Could you check a few things on this model? Use its own coordinates, in mm. Give positions to 0.01 mm unless a question says otherwise; leave off trailing zeros. Write each loop counter-clockwise with the first axis right and the second up, starting at its lowest first coordinate (ties: lowest second). Pieces come first, ordered by that corner, then holes. Notation, with made-up numbers: (85, 32) -> (99, 32) arc R13 cw to (99, 37) -> close; hole circle Ø7 at (-19, 19.25). An arc over 180 degrees is marked (long way). One line per question, with ' | ' between items.
from build123d import *

# Parameters (mm, degrees)
CYLINDER1271_R     = 1.5
CYLINDER1271_DEPTH = 100
CYLINDER1270_R     = 1.5
CYLINDER1270_DEPTH = 100
CYLINDER1269_R     = 1.5
CYLINDER1269_DEPTH = 32
CYLINDER1268_R     = 1.5
CYLINDER1268_DEPTH = 32
BOX235_W           = 200
BOX235_H           = 100
BOX235_DEPTH       = 100
BOX233_W           = 200
BOX233_H           = 100
BOX233_DEPTH       = 100
CYLINDER1127_R     = 4
CYLINDER1127_DEPTH = 100
CYLINDER1128_R     = 4
CYLINDER1128_DEPTH = 100
CYLINDER1129_R     = 4
CYLINDER1129_DEPTH = 100
CYLINDER1125_R     = 4
CYLINDER1125_DEPTH = 100
CYLINDER1130_R     = 4
CYLINDER1130_DEPTH = 100
CYLINDER1126_R     = 4
CYLINDER1126_DEPTH = 100
CYLINDER1102_R     = 1.5
CYLINDER1102_DEPTH = 100
CYLINDER1103_R     = 1.5
CYLINDER1103_DEPTH = 100
CYLINDER1104_R     = 1.5
CYLINDER1104_DEPTH = 100
CYLINDER1105_R     = 1.5
CYLINDER1105_DEPTH = 100
CYLINDER1106_R     = 1.5
CYLINDER1106_DEPTH = 100
CYLINDER1107_R     = 1.5
CYLINDER1107_DEPTH = 100
CYLINDER1108_R     = 1.5
CYLINDER1108_DEPTH = 100
CYLINDER1101_R     = 1.5
CYLINDER1101_DEPTH = 100
CYLINDER1092_R     = 59
CYLINDER1092_DEPTH = 4


with BuildPart() as obj1:
    # Cylinder1271 → Cylinder1271 (new body)
    with BuildSketch(Plane(origin=(14, 0, -60), x_dir=(1, 0, 0), z_dir=(0, 0, 1))):
        Circle(CYLINDER1271_R)
    extrude(amount=CYLINDER1271_DEPTH)


with BuildPart() as obj2:
    # Cylinder1270 → Cylinder1270 (new body)
    with BuildSketch(Plane(origin=(90, 0, -60), x_dir=(1, 0, 0), z_dir=(0, 0, 1))):
        Circle(CYLINDER1270_R)
    extrude(amount=CYLINDER1270_DEPTH)

    # Compound834: union obj1
    add(obj1.part)


with BuildPart() as obj3:
    # Cylinder1269 → Cylinder1269 (new body)
    with BuildSketch(Plane(origin=(78, 41, -42), x_dir=(1, 0, 0), z_dir=(0, 0, 1))):
        Circle(CYLINDER1269_R)
    extrude(amount=CYLINDER1269_DEPTH)


with BuildPart() as compound833:
    # Cylinder1268 → Cylinder1268 (new body)
    with BuildSketch(Plane(origin=(26, 41, -42), x_dir=(1, 0, 0), z_dir=(0, 0, 1))):
        Circle(CYLINDER1268_R)
    extrude(amount=CYLINDER1268_DEPTH)

    # Compound833: union obj3
    add(obj3.part)


with BuildPart() as krychle235:
    # Box235 → Box235 (new body)
    with BuildSketch(Plane(origin=(-60, 44, -90), x_dir=(1, 0, 0), z_dir=(0, 0, 1))):
        with Locations((100, 50)):
            Rectangle(BOX235_W, BOX235_H)
    extrude(amount=BOX235_DEPTH)


with BuildPart() as krychle233:
    # Box233 → Box233 (new body)
    with BuildSketch(Plane(origin=(-60, -144, -90), x_dir=(1, 0, 0), z_dir=(0, 0, 1))):
        with Locations((100, 50)):
            Rectangle(BOX233_W, BOX233_H)
    extrude(amount=BOX233_DEPTH)


with BuildPart() as obj4:
    # Cylinder1127 → Cylinder1127 (new body)
    with BuildSketch(Plane(origin=(-36, 34, -90), x_dir=(1, 0, 0), z_dir=(0, 0, 1))):
        Circle(CYLINDER1127_R)
    extrude(amount=CYLINDER1127_DEPTH)


with BuildPart() as obj5:
    # Cylinder1128 → Cylinder1128 (new body)
    with BuildSketch(Plane(origin=(-36, -34, -90), x_dir=(1, 0, 0), z_dir=(0, 0, 1))):
        Circle(CYLINDER1128_R)
    extrude(amount=CYLINDER1128_DEPTH)


with BuildPart() as obj6:
    # Cylinder1129 → Cylinder1129 (new body)
    with BuildSketch(Plane(origin=(50, 0, -90), x_dir=(1, 0, 0), z_dir=(0, 0, 1))):
        Circle(CYLINDER1129_R)
    extrude(amount=CYLINDER1129_DEPTH)


with BuildPart() as obj7:
    # Cylinder1125 → Cylinder1125 (new body)
    with BuildSketch(Plane(origin=(36, 34, -90), x_dir=(1, 0, 0), z_dir=(0, 0, 1))):
        Circle(CYLINDER1125_R)
    extrude(amount=CYLINDER1125_DEPTH)


with BuildPart() as obj8:
    # Cylinder1130 → Cylinder1130 (new body)
    with BuildSketch(Plane(origin=(36, -34, -90), x_dir=(1, 0, 0), z_dir=(0, 0, 1))):
        Circle(CYLINDER1130_R)
    extrude(amount=CYLINDER1130_DEPTH)


with BuildPart() as obj9:
    # Cylinder1126 → Cylinder1126 (new body)
    with BuildSketch(Plane(origin=(-50, 0, -90), x_dir=(1, 0, 0), z_dir=(0, 0, 1))):
        Circle(CYLINDER1126_R)
    extrude(amount=CYLINDER1126_DEPTH)

    # Compound565: union obj4, obj5, obj6, obj7, obj8
    add(obj4.part)
    add(obj5.part)
    add(obj6.part)
    add(obj7.part)
    add(obj8.part)


with BuildPart() as obj10:
    # Cylinder1102 → Cylinder1102 (new body)
    with BuildSketch(Plane(origin=(103, 6, -60), x_dir=(1, 0, 0), z_dir=(0, 0, 1))):
        Circle(CYLINDER1102_R)
    extrude(amount=CYLINDER1102_DEPTH)


with BuildPart() as obj11:
    # Cylinder1103 → Cylinder1103 (new body)
    with BuildSketch(Plane(origin=(76, 18, -60), x_dir=(1, 0, 0), z_dir=(0, 0, 1))):
        Circle(CYLINDER1103_R)
    extrude(amount=CYLINDER1103_DEPTH)


with BuildPart() as obj12:
    # Cylinder1104 → Cylinder1104 (new body)
    with BuildSketch(Plane(origin=(91, -21, -60), x_dir=(1, 0, 0), z_dir=(0, 0, 1))):
        Circle(CYLINDER1104_R)
    extrude(amount=CYLINDER1104_DEPTH)


with BuildPart() as obj13:
    # Cylinder1105 → Cylinder1105 (new body)
    with BuildSketch(Plane(origin=(13, -21, -60), x_dir=(1, 0, 0), z_dir=(0, 0, 1))):
        Circle(CYLINDER1105_R)
    extrude(amount=CYLINDER1105_DEPTH)


with BuildPart() as obj14:
    # Cylinder1106 → Cylinder1106 (new body)
    with BuildSketch(Plane(origin=(28, 18, -60), x_dir=(1, 0, 0), z_dir=(0, 0, 1))):
        Circle(CYLINDER1106_R)
    extrude(amount=CYLINDER1106_DEPTH)


with BuildPart() as obj15:
    # Cylinder1107 → Cylinder1107 (new body)
    with BuildSketch(Plane(origin=(1, -12, -60), x_dir=(1, 0, 0), z_dir=(0, 0, 1))):
        Circle(CYLINDER1107_R)
    extrude(amount=CYLINDER1107_DEPTH)


with BuildPart() as obj16:
    # Cylinder1108 → Cylinder1108 (new body)
    with BuildSketch(Plane(origin=(1, 6, -60), x_dir=(1, 0, 0), z_dir=(0, 0, 1))):
        Circle(CYLINDER1108_R)
    extrude(amount=CYLINDER1108_DEPTH)


with BuildPart() as obj17:
    # Cylinder1101 → Cylinder1101 (new body)
    with BuildSketch(Plane(origin=(103, -12, -60), x_dir=(1, 0, 0), z_dir=(0, 0, 1))):
        Circle(CYLINDER1101_R)
    extrude(amount=CYLINDER1101_DEPTH)

    # Compound562: union obj10, obj11, obj12, obj13, obj14, obj15, obj16
    add(obj10.part)
    add(obj11.part)
    add(obj12.part)
    add(obj13.part)
    add(obj14.part)
    add(obj15.part)
    add(obj16.part)


with BuildPart() as cut291:
    # Cylinder1092 → Cylinder1092 (new body)
    with BuildSketch(Plane(origin=(52, 0, -26), x_dir=(1, 0, 0), z_dir=(0, 0, 1))):
        Circle(CYLINDER1092_R)
    extrude(amount=CYLINDER1092_DEPTH)

    # Cut250: cut obj17
    add(obj17.part, mode=Mode.SUBTRACT)

    # Cut251: cut obj9
    add(obj9.part, mode=Mode.SUBTRACT)

    # Cut285: cut Krychle233
    add(krychle233.part, mode=Mode.SUBTRACT)

    # Cut287: cut Krychle235
    add(krychle235.part, mode=Mode.SUBTRACT)

    # Cut288: cut Compound833
    add(compound833.part, mode=Mode.SUBTRACT)

    # Cut291: cut obj2
    add(obj2.part, mode=Mode.SUBTRACT)


solid = cut291.part
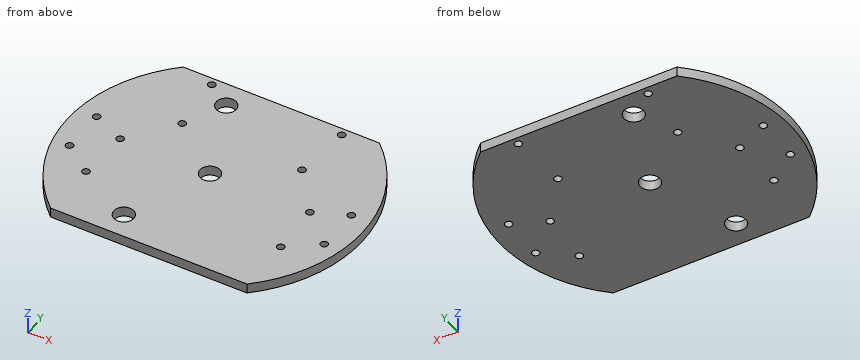
Q1. Imagine slicing it at A-A on y = 0. Please give me the cut outline in (x, z), and give its area (3 significant figures).
Answer below:
outline: (-7, -26) -> (12.5, -26) -> (12.5, -22) -> (-7, -22) -> close; (15.5, -26) -> (46, -26) -> (46, -22) -> (15.5, -22) -> close; (54, -26) -> (88.5, -26) -> (88.5, -22) -> (54, -22) -> close; (91.5, -26) -> (111, -26) -> (111, -22) -> (91.5, -22) -> close | area: 416 mm^2
Q2. If I drill on line 1 along Y through (x, z) = (36, -24.1); line 2 along X through (y, z) = (-21, -24); line 3 along X through (y, z) = (6, -25.2), over which ranges is the centre line in solid material (lowest first)?
Answer below:
line 1: y = -44 to -38, -30 to 30, 38 to 44 | line 2: x = -3.14 to 11.5, 14.5 to 89.5, 92.5 to 107.14 | line 3: x = -6.69 to -0.5, 2.5 to 101.5, 104.5 to 110.69
Q3. Will this pin go through, and if not, where does the flat tip stop? pin 1 (3.5 mm diameter, centred on x = 1, y = -12, fed in from +Z).
Answer below:
pin 1: stops at z = -22
Q4. Imagine slicing it at D-D on y = -21. Please give me the cut outline in (x, z).
Answer below:
outline: (-3.14, -26) -> (11.5, -26) -> (11.5, -22) -> (-3.14, -22) -> close; (14.5, -26) -> (89.5, -26) -> (89.5, -22) -> (14.5, -22) -> close; (92.5, -26) -> (107.14, -26) -> (107.14, -22) -> (92.5, -22) -> close
Q5. Imagine slicing it at C-C on z = -23.15. Count the separate pieces of the cut face and the enclosed holes in it, and give its area (3 significant figures).
Answer below:
separate pieces: 1 | enclosed holes: 15 | area: 9,080 mm^2
Q6. Imagine slicing it at B-B on x = 1. Please give me the cut outline in (y, z), and give its area (3 significant figures).
Answer below:
outline: (-29.66, -26) -> (-13.5, -26) -> (-13.5, -22) -> (-29.66, -22) -> close; (-10.5, -26) -> (4.5, -26) -> (4.5, -22) -> (-10.5, -22) -> close; (7.5, -26) -> (29.66, -26) -> (29.66, -22) -> (7.5, -22) -> close | area: 213 mm^2
